Part model, mm, in its own coordinate system. A direction names the side the tool comes from. Round coordinates to 2 decimals unless told otherwise and drop trailing zeros. Write each loop counter-clockwise with the first axis right and the second up, starting at its lowest first coordinate (ties: lowest second). Pieces come first, ordered by that corner, then holes. Notation, with made-up numbers: M -21,-6 L -14,-6 A11 cw -14,7 Z; hole C 63.5,38.25 d4. An arc over 180 degrees is marked long. Use a Markdown table: item, result. Add a question column.
1) Drop flat-ended pins along their axis: P1, Ø1, axis at x = 6, y = 74, coming from the +Z side; P2, Ø5, axis at x = 4, y = 41, coming from the +Z side; P3, Ø5, axis at x = 4.5, y = 88.5, coming from the +Z side. Give the stop position or say it passes through.
2) Wall check: probe 1 along Y at (x, z) = (1.25, 53.5); probe 2 along Y at (x, z) = (1.25, 114); probe 3 along Y at (x, z) = (3.75, 11). Give the ranges that are in metal, low to high.
3) Slice it at D-D on z = 46.5. Write the cut outline in (x, y).
4) Slice it at C-C on x = 4.5. Write the cut outline in (y, z), plus the area to 3 significant figures.
5) Slice it at A-A on z = 123.5. Write the cut outline in (x, y), plus the area to 3 significant figures.
6) Two-plate mould, pull along Y, no slides. Class faces 1 (the face through (7.4, 28.61, 127.59)), 2 (the face through (7, 0, 154)), 3 (the face through (7.395, 57.173, 119.796)): released by +Y, released by -Y, zero draft, split by the parting line, or undercut.
7) Which spindle directions (+Z, -Z, +X, -X, +Y, -Y) get a long thin tool onto all of the face, cutting with end or side? Do faces 4 (the face through (7, 50, 65)), 5 (the face through (7.395, 7.656, 168.428)), 6 (the face through (7.4, 29.59, 3.61)). Say none if no direction does.
8) Slice it at B-B on y = 10.5. Write the cut outline in (x, z).
Autodesk Inventor part; units mm, degrees
ref_plane "YZ Plane" through (0, 0, 0) normal (1, 0, 0) x (0, 1, 0)
ref_plane "XZ Plane" through (0, 0, 0) normal (0, 1, 0) x (-1, 0, 0)
ref_plane "XY Plane" through (0, 0, 0) normal (0, 0, 1) x (1, 0, 0)
sketch "Sketch2" plane through (0, 0, 0) normal (1, 0, 0) x (0, 1, 0)
  line L0 (0, 0) -> (100, 0)
  line L1 (100, 0) -> (100, 100)
  line L2 (0, 0) -> (0, 197) construction
  line L3 (0, 197) -> (15.5291, 139.0445)
  line L4 (0, 197) -> (60, 197) construction
  line L5 (15.5291, 139.0445) -> (100, 100)
  line L6 (0, 0) -> (24, 0) construction
  line L7 (24, 0) -> (24, 29) construction
  line L8 (24, 29) -> (0, 29) construction
  line L9 (0, 29) -> (0, 0) construction
  line L10 (24, 29) -> (24, 102) construction
  arc A0 (0, 19) -> (50, 29) centre (24, 29) ccw
  line L11 (0, 0) -> (0, 19)
  arc A1 (50, 102) -> (0, 112) centre (24, 102) ccw
  line L12 (24, 102) -> (50, 102) construction
  line L13 (24, 29) -> (50, 29) construction
  line L14 (50, 29) -> (50, 102)
  line L15 (0, 112) -> (0, 197)
  dimension "d10" = 100
  dimension "d11" = 100
  dimension "d12" = 197
  dimension "d13" = 60
  dimension "d14" = 75
  dimension "d15" = 24
  dimension "d16" = 29
  dimension "d17" = 73
  dimension "d18" = 26
  dimension "d19" = 26
extrude "Extrusion1" add sketch "Sketch2" along normal blind 15
properties part number "Side Plate"
Entries:
| question | item | result |
|---|---|---|
| 1 | P1 | stops at z = 112.25 |
| 1 | P2 | stops at z = 128.43 |
| 1 | P3 | stops at z = 106.47 |
| 2 | probe 1 | y = 50 to 100 |
| 2 | probe 2 | y = 0 to 0.93, 47.07 to 69.71 |
| 2 | probe 3 | y = 0 to 5.24, 42.76 to 100 |
| 3 | outline | M 0,50 L 15,50 L 15,100 L 0,100 Z |
| 4 | outline | M 0,0 L 100,0 L 100,100 L 15.53,139.04 L 0,197 L 0,112 A26 cw 50,102 L 50,29 A26 cw 0,19 Z |
| 4 | area | 6,960 mm^2 |
| 5 | outline | M 0,0 L 15,0 L 15,9.38 L 0,9.38 Z; M 0,38.62 L 15,38.62 L 15,49.16 L 0,49.16 Z |
| 5 | area | 299 mm^2 |
| 6 | face 1 | undercut |
| 6 | face 2 | released by -Y |
| 6 | face 3 | released by +Y |
| 7 | face 4 | +X, -X, -Y |
| 7 | face 5 | +Z, +X, -X, +Y |
| 7 | face 6 | +X, -X |
| 8 | outline | M 0,0 L 15,0 L 15,6.78 L 0,6.78 Z; M 0,124.22 L 15,124.22 L 15,157.81 L 0,157.81 Z |
